The figure shows three views and two pictorial views of one solid part (mm, origin at its lowest corner). Answer the questions. A direction names the side the tool comes from. Coordinates: 2 decimals unless noted, no trailing zeros. Write each loop counter-clockwise with the first axis right and the second up, starting at its lowest first coordinate (ties: lowest second). Pieces come first, ordered by that corner, then holes.
Item 1: Straight lines are drawn through the part: probe 1 along Z at (x, y) = (12.7, 24.55); probe 2 along X at (y, z) = (2.5, 23) (1 decimal); probe 3 along Y at (x, z) = (3, 20.5) (1 decimal). For each, find the intervals that lie inside material, in ascending order.
Item 2: Section B-B (y = 12.7) is taken. Give the vertices of the cut face in (x, z) (1 decimal).
Item 3: Each of these flat-tipped pins is pushed along its axis until it touches: P1, Ø6, axis at x = 16.5, z = 12, coming from the -Y side (3 decimals); P2, Ø8, axis at y = 12.7, z = 31.75, coming from the +X side (3 decimals). Where does it stop, or does it pass through?
Item 4: Section D-D (z = 15) is taken. Give the vertices of the cut face in (x, y) (1 decimal).
Item 5: Section C-C (z = 31.75) is taken. Give the vertices of the cut face in (x, y) (1 decimal), then the cut area to 3 significant figures.
Item 6: A tool of negligible diameter and unlimited length cuts with its end or side. For the marked faces 1 and 2, from which of +Z, -Z, +X, -X, +Y, -Y can it reach the whole face along a straight path? Write none if from no direction.
Item 7: Section A-A (x = 12.7) is taken. Give the vertices of the cut face in (y, z) (1 decimal).
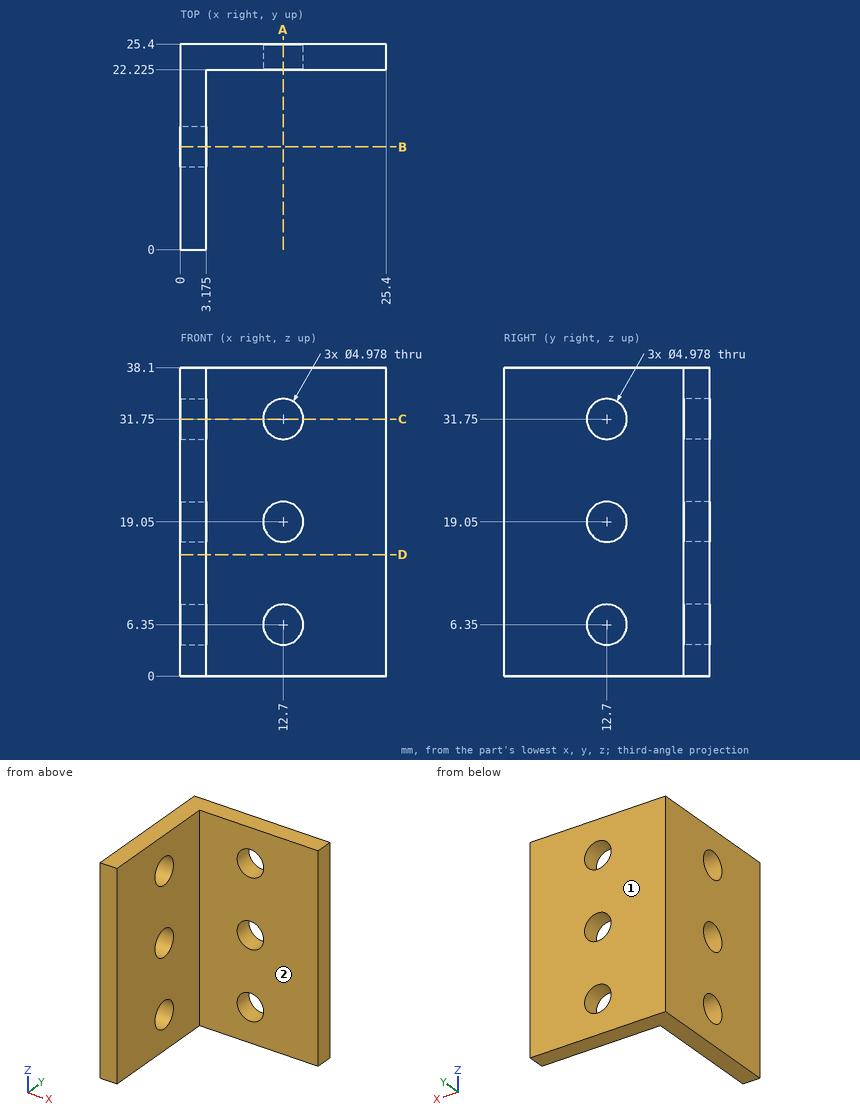
Established:
1. probe 1: z = 0 to 3.86, 8.84 to 16.56, 21.54 to 29.26, 34.24 to 38.1
1. probe 2: x = 0 to 3.2
1. probe 3: y = 0 to 10.7, 14.7 to 25.4
2. outline: (0, 0) - (3.2, 0) - (3.2, 3.9) - (0, 3.9) - close; (0, 8.8) - (3.2, 8.8) - (3.2, 16.6) - (0, 16.6) - close; (0, 21.5) - (3.2, 21.5) - (3.2, 29.3) - (0, 29.3) - close; (0, 34.2) - (3.2, 34.2) - (3.2, 38.1) - (0, 38.1) - close
3. P1: stops at y = 22.225
3. P2: stops at x = 3.175
4. outline: (0, 0) - (3.2, 0) - (3.2, 22.2) - (25.4, 22.2) - (25.4, 25.4) - (0, 25.4) - close
5. outline: (0, 0) - (3.2, 0) - (3.2, 10.2) - (0, 10.2) - close; (0, 15.2) - (3.2, 15.2) - (3.2, 22.2) - (10.2, 22.2) - (10.2, 25.4) - (0, 25.4) - close; (15.2, 22.2) - (25.4, 22.2) - (25.4, 25.4) - (15.2, 25.4) - close
5. area: 120 mm2
6. face 1: +Z, -Z, +X, -X, +Y
6. face 2: +Z, -Z, +X, -Y
7. outline: (22.2, 0) - (25.4, 0) - (25.4, 3.9) - (22.2, 3.9) - close; (22.2, 8.8) - (25.4, 8.8) - (25.4, 16.6) - (22.2, 16.6) - close; (22.2, 21.5) - (25.4, 21.5) - (25.4, 29.3) - (22.2, 29.3) - close; (22.2, 34.2) - (25.4, 34.2) - (25.4, 38.1) - (22.2, 38.1) - close
